The model under review builds one solid part; all positions refer to its coordinate system, in mm. Face numbers are marked on the shaded views. A direction names the side the tool comes from. Give positions to 0.01 mm unless a question says otherwise; leave off trailing zeros. Order: outer loops, then holes, each group sorted by start corner. A loop starts at its lowest first (then second) coordinate and runs counter-clockwise, first axis right, second up. Notation, with made-up numbers: (-32, 10.5) - (10, 10.5) arc R32 ccw to (10, 43.5) - close; hole circle Ø8 at (37, 84). An arc over 180 degrees is marked (long way). Put each result on its own line as item: value.
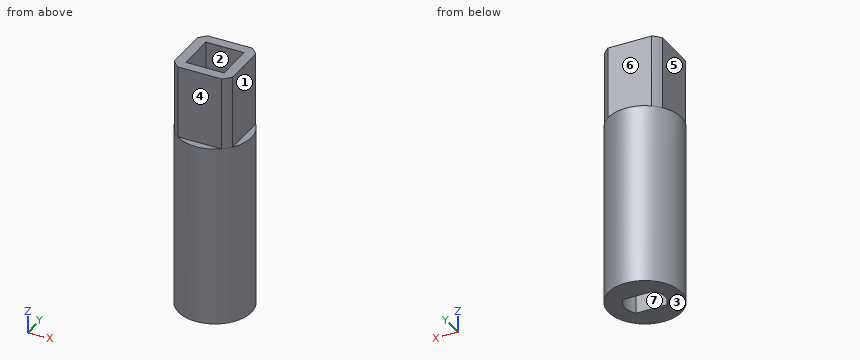
```python
from build123d import *

# Parameters (mm, degrees)
SKETCH1_R           = 5
BOSS_EXTRUDE1_DEPTH = 25
CUT_EXTRUDE1_DEPTH  = 9.3
BOSS_EXTRUDE2_DEPTH = 10
SKETCH4_W           = 5.25
SKETCH4_H           = 5.25
CUT_EXTRUDE2_DEPTH  = 10


with BuildPart() as part:
    # Sketch1 → Boss-Extrude1 (new body)
    with BuildSketch(Plane.XY):
        Circle(SKETCH1_R)
    extrude(amount=BOSS_EXTRUDE1_DEPTH)

    # Sketch2 → Cut-Extrude1 (cut)
    with BuildSketch(Plane(origin=(0, 0, 0), x_dir=(-1, 0, 0), z_dir=(0, 0, -1))):
        with BuildLine():
            Line((-2.112335797, -1.727538634), (2.13030489, -1.727538634))
            ThreePointArc((2.13030489, -1.727538634), (2.758984546, 0.022461366), (2.13030489, 1.772461366))
            Line((2.13030489, 1.772461366), (-2.112335797, 1.772461366))
            ThreePointArc((-2.112335797, 1.772461366), (-2.741015454, 0.022461366), (-2.112335797, -1.727538634))
        make_face()
    extrude(amount=-CUT_EXTRUDE1_DEPTH, mode=Mode.SUBTRACT)

    # Sketch3 → Boss-Extrude2 (add)
    with BuildSketch(Plane.XY.offset(25)):
        with BuildLine():
            ThreePointArc((-4, -3), (-3.535533906, -3.535533906), (-3, -4))
            Line((-3, -4), (3, -4))
            ThreePointArc((3, -4), (3.535533906, -3.535533906), (4, -3))
            Line((4, -3), (4, 3))
            ThreePointArc((4, 3), (3.535533906, 3.535533906), (3, 4))
            Line((3, 4), (-3, 4))
            ThreePointArc((-3, 4), (-3.535533906, 3.535533906), (-4, 3))
            Line((-4, 3), (-4, -3))
        make_face()
    extrude(amount=BOSS_EXTRUDE2_DEPTH)

    # Sketch4 → Cut-Extrude2 (cut)
    with BuildSketch(Plane.XY.offset(35)):
        Rectangle(SKETCH4_W, SKETCH4_H)
    extrude(amount=-CUT_EXTRUDE2_DEPTH, mode=Mode.SUBTRACT)


solid = part.part
```
(1) For the marked faces 1, 2, 3 and 4, list the 3-axis set-ups (+Z, -Z, +X, -X, +Y, -Y) from which the entire face can be reached by the end or side of a thin tool; tool diameter is ignored.
The answers:
face 1: +Z, +X, +Y, -Y
face 2: +Z
face 3: -Z, +X, -X, +Y, -Y
face 4: +Z, +X, -X, -Y
(2) Take a section at C-C, the plane y = 0. Write out the cut boundary in (x, z) (3 decimals).
The answers:
outline: (-5, 0) - (-2.759, 0) - (-2.759, 9.3) - (2.741, 9.3) - (2.741, 0) - (5, 0) - (5, 25) - (4, 25) - (4, 35) - (2.625, 35) - (2.625, 25) - (-2.625, 25) - (-2.625, 35) - (-4, 35) - (-4, 25) - (-5, 25) - close
(3) Clearance check with flat-ended pins moving along their axes: pin 1 Ø1.6 at (x, y) = (-0.5, 0) entering from +Z; pin 2 Ø1 at (x, y) = (0, 0.5) entering from -Z; pin 3 Ø2.5 at (y, z) = (0.5, 27.5) entering from +X; pin 4 Ø1.1 at (x, y) = (-1, -4.5) entering from +Z. State where each tip first meets the part, or that it passes through.
The answers:
pin 1: z = 25
pin 2: z = 9.3
pin 3: x = 4
pin 4: z = 35
(4) The part is to be moulded in two halves that separate along Y. For the marked faces 5, 6 and 7, say which applies: pulls with the +Y half, pulls with the -Y half, needs draft (parallel to the pull), parting line crosses it, or undercut.
The answers:
face 5: needs draft
face 6: pulls with the +Y half
face 7: undercut
(5) Wall thickness on L1, parallel to Y at x = -2.25, z = 31.5 (3 decimals); L2, parallel to Z at x = 1.5, y = 0: over which ranges is each line inside the solid? List them lowest first.
The answers:
L1: -4 to -2.625, 2.625 to 4
L2: 9.3 to 25
(6) Take a section at A-A, the plane z = 4. Write out the cut boundary in (x, y), then the cut area to 3 significant figures.
The answers:
outline: circle Ø10 at (0, 0); hole (-2.13, -1.73) - (2.11, -1.73) arc R2.75 ccw to (2.11, 1.77) - (-2.13, 1.77) arc R2.75 ccw to start
area: 60.7 mm^2
(7) Take a section at D-D, the plane z = 29.5. Write out the cut boundary in (x, y) (3 decimals), then the cut area to 3 significant figures.
The answers:
outline: (-4, -3) arc R5 ccw to (-3, -4) - (3, -4) arc R5 ccw to (4, -3) - (4, 3) arc R5 ccw to (3, 4) - (-3, 4) arc R5 ccw to (-4, 3) - close; hole (-2.625, -2.625) - (2.625, -2.625) - (2.625, 2.625) - (-2.625, 2.625) - close
area: 34.6 mm^2
(8) Take a section at B-B, the plane x = 0. Write out the cut boundary in (y, z) (3 decimals).
The answers:
outline: (-5, 0) - (-1.728, 0) - (-1.728, 9.3) - (1.772, 9.3) - (1.772, 0) - (5, 0) - (5, 25) - (4, 25) - (4, 35) - (2.625, 35) - (2.625, 25) - (-2.625, 25) - (-2.625, 35) - (-4, 35) - (-4, 25) - (-5, 25) - close
